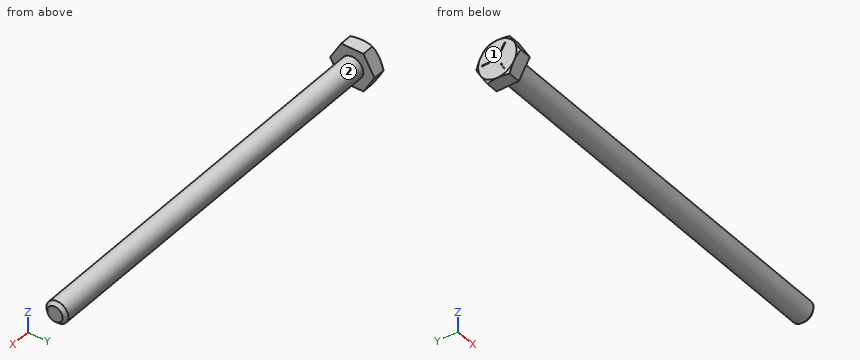
```python
from build123d import *

# Parameters (mm, degrees)
SKETCH5_R           = 3.175
BOSS_EXTRUDE3_DEPTH = 114.3
CHAMFER1_SIZE       = 0.9525
BOSS_EXTRUDE4_DEPTH = 3.96875
SKETCH8_OUTSIDE_W   = 450.168
SKETCH8_OUTSIDE_H   = 451.888
SKETCH8_OUTSIDE_R   = 5.55625
CUT_EXTRUDE3_DEPTH  = 119.26875
CUT_EXTRUDE3_TAPER  = 60
CUT_EXTRUDE4_DEPTH  = 0.254
CIRPATTERN1_COUNT   = 3


with BuildPart() as part:
    # Sketch5 → Boss-Extrude3 (new body)
    with BuildSketch(Plane(origin=(59.134375, 0, 0), x_dir=(0, 0, -1), z_dir=(1, 0, 0))):
        Circle(SKETCH5_R)
    extrude(amount=-BOSS_EXTRUDE3_DEPTH)

    # Chamfer1
    chamfer1_edges = [part.edges().sort_by_distance(p)[0] for p in [
        (59.134375, 0, 3.175),
    ]]
    chamfer(chamfer1_edges, length=CHAMFER1_SIZE)

    # Sketch11 → Revolve1 (revolve)
    with BuildSketch(Plane.XY):
        Polygon((-55.165625, 3.175), (-55.165625, 0), (43.259375, 0), (40.084375, 3.175), align=None)
    revolve(axis=Axis((-55.165625, 0, 0), (1, 0, 0)))

    # Sketch6 → Boss-Extrude4 (add)
    with BuildSketch(Plane.ZY.offset(55.165625)):
        Polygon((5.55625, 3.207902433), (0, 6.415804866), (-5.55625, 3.207902433), (-5.55625, -3.207902433), (0, -6.415804866), (5.55625, -3.207902433), align=None)
    extrude(amount=BOSS_EXTRUDE4_DEPTH)

    # Sketch8 outside → Cut-Extrude3 (cut, through all)
    with BuildSketch(Plane.ZY.offset(59.134375)):
        Rectangle(SKETCH8_OUTSIDE_W, SKETCH8_OUTSIDE_H)
        Circle(SKETCH8_OUTSIDE_R, mode=Mode.SUBTRACT)
    extrude(amount=-CUT_EXTRUDE3_DEPTH, taper=CUT_EXTRUDE3_TAPER, mode=Mode.SUBTRACT)

    # Sketch12 → Cut-Extrude4 (cut)
    with BuildSketch(Plane.ZY.offset(59.134375)):
        with BuildLine():
            Line((0.1666875, 4.2783125), (0.1666875, 2.3891875))
            ThreePointArc((0.1666875, 2.3891875), (0, 2.2225), (-0.1666875, 2.3891875))
            Line((-0.1666875, 2.3891875), (-0.1666875, 4.2783125))
            ThreePointArc((-0.1666875, 4.2783125), (0, 4.445), (0.1666875, 4.2783125))
        make_face()
    cut_extrude4 = extrude(amount=-CUT_EXTRUDE4_DEPTH, mode=Mode.SUBTRACT)

    # CirPattern1: Cut-Extrude4 ×3 about axis
    cirpattern1_axis = Axis((0, 0, 0), (1, 0, 0))
    for i in range(1, CIRPATTERN1_COUNT):
        add(cut_extrude4.rotate(cirpattern1_axis, i * 360 / CIRPATTERN1_COUNT), mode=Mode.SUBTRACT)


solid = part.part
```
Geometry: final body of the model. Coordinates: model frame, mm. Face numbers are marked on the shaded views. A direction names the side the tool comes from. Coordinates: 2 decimals unless noted, no trailing zeros. Order: outer loops, then holes, each group sorted by start corner. A loop starts at its lowest first (then second) coordinate and runs counter-clockwise, first axis right, second up. Notation, with made-up numbers: M 67.25,-10 L 103.25,-10 A27 ccw 103.25,17 Z; hole C 39.25,0.25 d5. An arc over 180 degrees is marked long. Answer in a Markdown table with one row per item. Add a question column.
Q1. Reachability of the marked faces 1 and 2 from +Z, -Z, +X, -X, +Y, -Y: full face, straight path, thin tool, end or side. Return the list, or none.
Q2. Contact query for a flat-ended pin moving along its axis: P1, Ø6, axis at x = -32, z = -2.5, coming from the +Y side (3 decimals). Output: stop coordinate, or through.
Q3. Section query A-A on x = 19. Return the cut outline in (y, z) (3 decimals).
Q4. Line query: L1, parallel to X at y = 0.75, z = 4.5; L2, parallel to Y at x = 54, z = -2.25; L3, parallel to Z at x = -1.5, y = -1.5. Output: solid intervals per line, ascending.
Completed:
| question | item | result |
|---|---|---|
| 1 | face 1 | +Z, -Z, -X, +Y, -Y |
| 1 | face 2 | +X |
| 2 | P1 | stops at y = 3.175 |
| 3 | outline | C 0,0 d6.35 |
| 4 | L1 | x = -59.13 to -55.17 |
| 4 | L2 | y = -2.24 to 2.24 |
| 4 | L3 | z = -2.8 to 2.8 |
